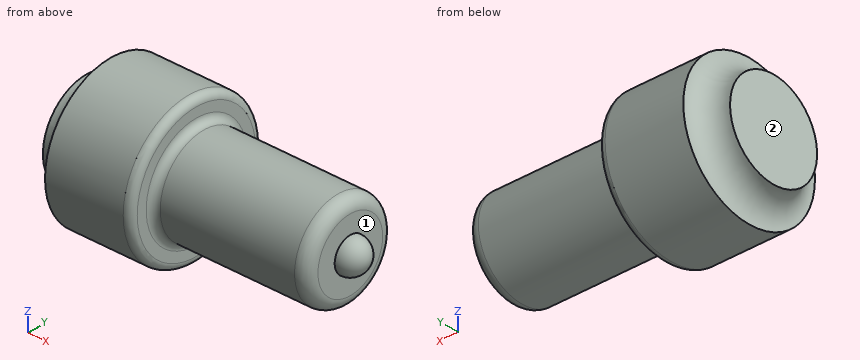
```python
from build123d import *


with BuildPart() as part:
    # Sketch1 → Revolve5 (revolve)
    with BuildSketch(Plane.XY):
        with BuildLine():
            Line((0, 0), (146.05, 0))
            ThreePointArc((146.05, 0), (143.446179285, 6.286179285), (137.16, 8.89))
            Line((137.16, 8.89), (137.16, 18.415))
            ThreePointArc((137.16, 18.415), (135.300128061, 22.905128061), (130.81, 24.765))
            Line((130.81, 24.765), (60.96, 24.765))
            ThreePointArc((60.96, 24.765), (58.265923164, 25.880923164), (57.15, 28.575))
            Line((57.15, 28.575), (57.15, 33.655))
            ThreePointArc((57.15, 33.655), (56.034076836, 36.349076836), (53.34, 37.465))
            Line((53.34, 37.465), (12.7, 37.465))
            ThreePointArc((12.7, 37.465), (8.980256121, 28.484743879), (0, 24.765))
            Line((0, 24.765), (0, 0))
        make_face()
    revolve(axis=Axis((0, 0, 0), (1, 0, 0)))


solid = part.part
```
Part model, mm, in its own coordinate system. Face numbers are marked on the shaded views. A direction names the side the tool comes from. Give positions to 0.01 mm unless a question says otherwise; leave off trailing zeros. Loops run counter-clockwise (first coordinate to the right, second up) from the corner with the lowest first, then second, coordinate; pieces in that order, holes last. Notation, with made-up numbers: M -17,37 L 37,37 A15 ccw 37,55 Z; hole C -28,0.5 d6. An arc over 180 degrees is marked long. Return JSON: item names as keys, results as strings.
1) Saw through at C-C, the plane x = 88. List the corners of the cut face in (y, z) (3 decimals), then the cut area to 3 significant figures.
Calculated:
{"outline": "C 0,0 d49.53", "area": "1,930 mm2"}
2) Drill centre lines: line 1 (X direction, y = 10, z = -15.5); line 2 (X direction, y = 17.5, z = 23); line 3 (Y direction, x = 24.5, z = 28). Where is each one in solid material? Low to high.
Calculated:
{"line 1": "x = 0 to 137.16", "line 2": "x = 9.38 to 57.15", "line 3": "y = -24.89 to 24.89"}
3) Saw through at D-D, the plane x = 17.5. List the corners of the cut face in (y, z) (3 decimals).
Calculated:
{"outline": "C 0,0 d74.93"}
4) Saw through at A-A, the plane z = 0. List the corners of the cut face in (x, y) (3 decimals).
Calculated:
{"outline": "M 0,-24.765 A12.7 cw 12.7,-37.465 L 53.34,-37.465 A3.81 ccw 57.15,-33.655 L 57.15,-28.575 A3.81 cw 60.96,-24.765 L 130.81,-24.765 A6.35 ccw 137.16,-18.415 L 137.16,-8.89 A8.89 ccw 137.16,8.89 L 137.16,18.415 A6.35 ccw 130.81,24.765 L 60.96,24.765 A3.81 cw 57.15,28.575 L 57.15,33.655 A3.81 ccw 53.34,37.465 L 12.7,37.465 A12.7 cw 0,24.765 Z"}
5) 3-axis set-ups, long thin cutter, end or side, ignore diameter. For the marked faces 1 and 2: which of +Z, -Z, +X, -X, +Y, -Y reach the whole face in a straight line?
Calculated:
{"face 1": "+X", "face 2": "+Z, -Z, -X, +Y, -Y"}
6) Flat gauge pins, fed straight in: pin 1 Ø5 at (y, z) = (27, -18) entering from -X; pin 2 Ø12 at (x, y) = (81, 27.5) entering from -Z; pin 3 Ø5 at (y, z) = (27, 21) entering from -X. Where does each tip first touch, or does it go through?
Calculated:
{"pin 1": "stops at x = 10.24", "pin 2": "stops at z = -12.29", "pin 3": "stops at x = 11.32"}
